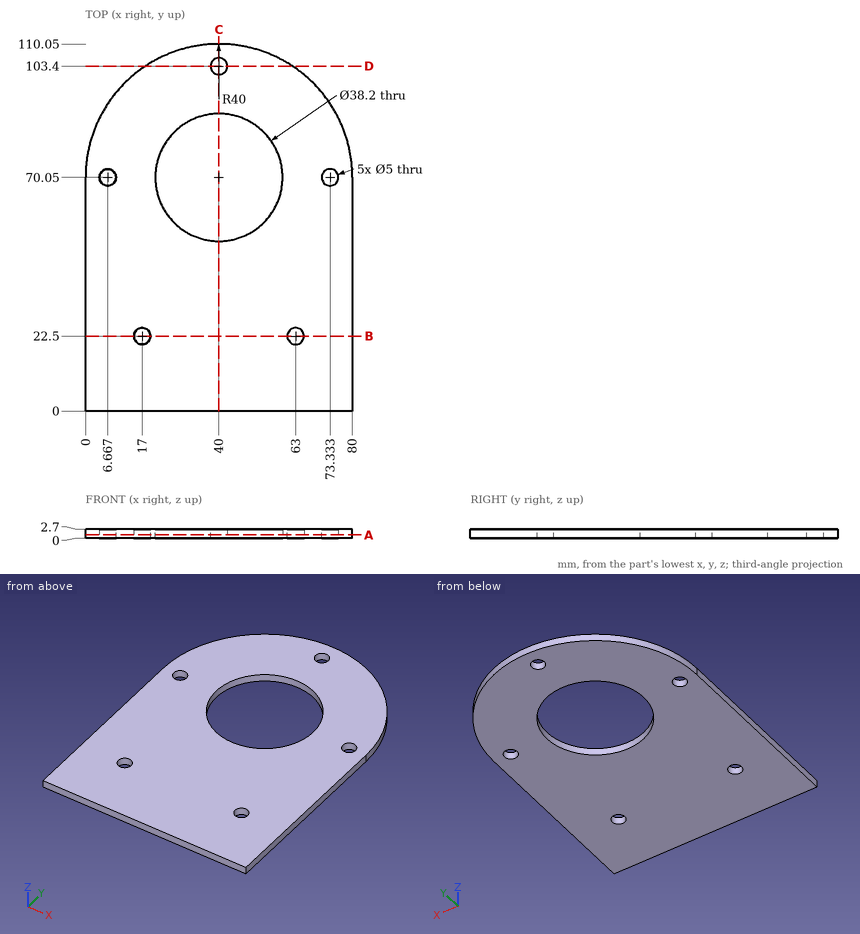
Study the drawing (mm; zero at the part's minimum x, y, z) and answer. Give positions to 0.01 mm unless a question says otherwise; leave off trailing zeros. Write each loop counter-clockwise with the first axis right and the second up, starting at its lowest first coordinate (ties: lowest second). Pieces come first, ordered by that corner, then holes. Notation, with made-up numbers: (-15, 16.5) - (23, 16.5) arc R35 ccw to (23, 52.5) - close; hole circle Ø1 at (44, 83.25). An arc over 180 degrees is marked (long way). Use CSV: the item, a comma, the result in double quotes. Start each with the question number.
(1) Consider line 1 along Y through (x, z) = (40, 1.25); line 2 along X through (y, z) = (21, 1.8); line 3 along Y through (x, z) = (15.5, 1.9). Determine where each line is inside the solid, lowest interval first.
(2) Find section A-A (z = 1). Give the vertices of the cut face in (x, y).
(3) Find section D-D (y = 103.4). Give the vertices of the cut face in (x, z).
(4) Find section B-B (y = 22.5). Give the vertices of the cut face in (x, z), plus the area to 3 significant figures.
(5) Find section C-C (x = 40). Give the vertices of the cut face in (y, z), plus the area to 3 significant figures.
(6) Given P1, Ø6, axis at x = 69, y = 16, coming from the -Z side; P2, Ø3, axis at x = 6.667, y = 70.05, coming from the +Z side, each flat-ended and moving along its own axis, determine where each tip first touches the part or whether it passes through.
Findings below:
1,line 1,"0 to 50.95, 89.15 to 100.9, 105.9 to 110.05"
1,line 2,"0 to 15, 19 to 61, 65 to 80"
1,line 3,"0 to 20.5, 24.5 to 101.67"
2,outline,"(0, 0) - (80, 0) - (80, 70.05) arc R40 ccw to (0, 70.05) - close; hole circle Ø5 at (6.67, 70.05); hole circle Ø5 at (17, 22.5); hole circle Ø38.2 at (40, 70.05); hole circle Ø5 at (40, 103.4); hole circle Ø5 at (63, 22.5); hole circle Ø5 at (73.33, 70.05)"
3,outline,"(17.91, 0) - (37.5, 0) - (37.5, 2.7) - (17.91, 2.7) - close; (42.5, 0) - (62.09, 0) - (62.09, 2.7) - (42.5, 2.7) - close"
4,outline,"(0, 0) - (14.5, 0) - (14.5, 2.7) - (0, 2.7) - close; (19.5, 0) - (60.5, 0) - (60.5, 2.7) - (19.5, 2.7) - close; (65.5, 0) - (80, 0) - (80, 2.7) - (65.5, 2.7) - close"
4,area,"189 mm2"
5,outline,"(0, 0) - (50.95, 0) - (50.95, 2.7) - (0, 2.7) - close; (89.15, 0) - (100.9, 0) - (100.9, 2.7) - (89.15, 2.7) - close; (105.9, 0) - (110.05, 0) - (110.05, 2.7) - (105.9, 2.7) - close"
5,area,"180 mm2"
6,P1,"z = 0"
6,P2,"through"
